```python
from build123d import *

# Parameters (mm, degrees)
CROQUIS1_W            = 530
CROQUIS1_H            = 450
CROQUIS1_W_2          = 520
CROQUIS1_H_2          = 440
EXTRUIR_L_MINA1_DEPTH = 50
CROQUIS2_W            = 530
CROQUIS2_H            = 450
EXTRUIR1_DEPTH        = 5


with BuildPart() as part:
    # Croquis1 → Extruir-Lámina1 (new body)
    with BuildSketch(Plane(origin=(0, 0, 0), x_dir=(1, 0, 0), z_dir=(0, 1, 0))):
        Rectangle(CROQUIS1_W, CROQUIS1_H)
        Rectangle(CROQUIS1_W_2, CROQUIS1_H_2, mode=Mode.SUBTRACT)
    extrude(amount=-EXTRUIR_L_MINA1_DEPTH)

    # Croquis2 → Extruir1 (add)
    with BuildSketch(Plane.XZ.offset(50)):
        Rectangle(CROQUIS2_W, CROQUIS2_H)
    extrude(amount=EXTRUIR1_DEPTH)


solid = part.part
```
Geometry: final body of the model. Coordinates: model frame, mm. A direction names the side the tool comes from. Give positions to 0.01 mm unless a question says otherwise; leave off trailing zeros. Loops run counter-clockwise (first coordinate to the right, second up) from the corner with the lowest first, then second, coordinate; pieces in that order, holes last. Notation, with made-up numbers: (4, 0) - (19, 0) arc R30 cw to (19, 31) - close; hole circle Ø7 at (-1, -14). An arc over 180 degrees is marked (long way). Answer as CSV lines item,"result". Start each with the question number.
(1) Reachability of faces 1 (the face through (-4, -25, -220)), 2 (the face through (265, -27, -3)) from +Z, -Z, +X, -X, +Y, -Y: full face, straight path, thin tool, end or side. Return the list, or none.
(2) Section query B-B (x = -137). Output: boundary loops of the cut face in (y, z).
(3) Ray query, line 1 along X through (y, z) = (-30.5, 15.5); line 2 along Z through (x, y) = (-163.5, -39); line 3 along Y through (x, z) = (147.5, -37.5). Return the intervals inside material, ascending. Write a range as [from, to].
(4) Section query A-A (z = 190). Output: boundary loops of the cut face in (x, y).
(5) Mould query, pull axis X, two halves, no side actions, for faces 3 (the face through (-4, -27, -225)), 4 (the face through (-260, -25, 3)), 5 (the face through (-265, -27, -3)). Classes: +X half, -X half, draft (parallel to the pull), parting line (faces both ways), or undercut.
(6) Section query C-C (y = -7.5). Output: boundary loops of the cut face in (x, z), and give its area (3 significant figures).
(7) Pin query (flat end, axial travel): P1, Ø1.5, axis at x = -178, z = -157.5, coming from the +Y side. Return the tip coordinate at first contact, or that it passes through.
Worked answers:
1,face 1,"+Y"
1,face 2,"+Z, -Z, +X, +Y, -Y"
2,outline,"(-55, -225) - (0, -225) - (0, -220) - (-50, -220) - (-50, 220) - (0, 220) - (0, 225) - (-55, 225) - close"
3,line 1,"x = [-265, -260], [260, 265]"
3,line 2,"z = [-225, -220], [220, 225]"
3,line 3,"y = [-55, -50]"
4,outline,"(-265, -55) - (265, -55) - (265, 0) - (260, 0) - (260, -50) - (-260, -50) - (-260, 0) - (-265, 0) - close"
5,face 3,"draft"
5,face 4,"undercut"
5,face 5,"-X half"
6,outline,"(-265, -225) - (265, -225) - (265, 225) - (-265, 225) - close; hole (-260, -220) - (260, -220) - (260, 220) - (-260, 220) - close"
6,area,"9,700 mm^2"
7,P1,"stops at y = -50"
